Read the model definition and answer for the solid it produces. Units are mm, in the model's axes. A direction names the side the tool comes from. Round coordinates to 2 decimals unless told otherwise and drop trailing zeros. Order: outer loops, then holes, each group sorted by start corner. A loop starts at its lowest first (then second) coordinate and runs counter-clockwise, first axis right, second up. Notation, with made-up numbers: (9, -7) -> (15, -7) arc R31 ccw to (15, 22) -> close; hole circle Ø7 at (79.25, -36). An arc over 180 degrees is marked (long way). One line per item, written item: value. Start each with the question number.
1. Consider line 1 (X direction, y = -10.5, z = 4.25); line 2 (Y direction, x = -12, z = 5); line 3 (Z direction, x = -15, y = 9.75). Determine where each line is inside the solid, lowest interval first.
2. Section B-B (y = -10) is taken. Give the vertices of the cut face in (x, z).
3. Section A-A (z = 4.75) is taken. State how many separate pieces and enclosed holes the cut face has, then the cut area to 3 significant figures.
4. Section C-C (x = -8) is taken. Give the vertices of the cut face in (y, z).
5. Flat-ended cylindrical pins translate along their axes: pin 1 Ø3 at (y, z) = (-9, 1.5) entering from +X; pin 2 Ø8 at (x, y) = (4.5, -2) entering from +Z. Find the tip coordinate at first contact, or state that the pin passes through.
6. For faces 1 (the face through (0, 14, 1)), 2 (the face through (-15.1, 7.675, 7.3)), 3 (the face through (-13.3, 0, 1)), determine the directions among +Z, -Z, +X, -X, +Y, -Y from which every point of the face is accessible in a straight line to the end or side of a thin tool.
7. The mould has two halves that part along X. Classify faces 4 (the face through (13, -2.217, 1)), 5 (the face through (0, -14, 1)): released by +X, released by -X, zero draft, split by the parting line, or undercut.
from build123d import *

# Parameters (mm, degrees)
F0_W     = 30
F0_H     = 28
F1_DEPTH = 1.5
F3_DEPTH = 28
F4_W     = 1.3
F4_H     = 4
F5_DEPTH = 25
F6_W     = 41.33358
F6_H     = 15.079705
F7_DEPTH = 25


with BuildPart() as f1:
    # F0 (on Top) → F1 (new body)
    with BuildSketch(Plane.XY):
        Rectangle(F0_W, F0_H)
    extrude(amount=F1_DEPTH)

    # F2 (on face) → F3 (join)
    with BuildSketch(Plane.XZ.offset(14)):
        with BuildLine():
            ThreePointArc((-11.75963, 1.5), (-11.010384, 2.78526), (-10.75, 4.25))
            ThreePointArc((-10.75, 4.25), (-18.005204, 7.255204), (-15, 0))
            Line((-15, 0), (-15, 1.5))
            Line((-15, 1.5), (-11.75963, 1.5))
        make_face()
        with BuildLine():
            ThreePointArc((-12.25, 4.25), (-13.055456, 2.305456), (-15, 1.5))
            ThreePointArc((-15, 1.5), (-16.944544, 6.194544), (-12.25, 4.25))
        make_face(mode=Mode.SUBTRACT)
        with BuildLine():
            Line((15, 1.5), (15, 0))
            ThreePointArc((15, 0), (18.005204, 1.244796), (19.25, 4.25))
            ThreePointArc((19.25, 4.25), (13.53526, 8.239616), (11.75963, 1.5))
            Line((11.75963, 1.5), (15, 1.5))
        make_face()
        with BuildLine():
            ThreePointArc((17.75, 4.25), (16.944544, 2.305456), (15, 1.5))
            ThreePointArc((15, 1.5), (13.055456, 6.194544), (17.75, 4.25))
        make_face(mode=Mode.SUBTRACT)
        with BuildLine():
            Line((-15, 1.5), (-15, 0))
            ThreePointArc((-15, 0), (-13.214643, 0.393188), (-11.75963, 1.5))
            Line((-11.75963, 1.5), (-15, 1.5))
        make_face()
    extrude(amount=-F3_DEPTH)

    # F4 (on face) → F5 (cut)
    with BuildSketch(Plane.XY.offset(1.5)):
        with Locations((-12.65, -0.217311)):
            Rectangle(F4_W, F4_H)
        with Locations((12.65, -0.217311)):
            Rectangle(F4_W, F4_H)
    extrude(amount=-F5_DEPTH, mode=Mode.SUBTRACT)

    # F6 (on face) → F7 (cut)
    with BuildSketch(Plane.XY.offset(1.5)):
        with Locations((0.027121, 0.135609)):
            Rectangle(F6_W, F6_H)
    extrude(amount=F7_DEPTH, mode=Mode.SUBTRACT)


solid = f1.part
Answer:
1. line 1: -19.25 to -17.75, -12.25 to -10.75, 10.75 to 12.25, 17.75 to 19.25
1. line 2: -14 to -7.4, 7.68 to 14
1. line 3: 0 to 1.5, 7 to 8.5
2. outline: (-15, 0) -> (15, 0) arc R4.25 ccw (long way) to (11.76, 1.5) -> (-11.76, 1.5) arc R4.25 ccw (long way) to start; hole (-15, 1.5) arc R2.75 ccw to (-12.25, 4.25) arc R2.75 ccw (long way) to start; hole (15, 1.5) arc R2.75 ccw to (17.75, 4.25) arc R2.75 ccw (long way) to start
3. separate pieces: 8
3. enclosed holes: 0
3. area: 78.4 mm^2
4. outline: (-14, 0) -> (14, 0) -> (14, 1.5) -> (-14, 1.5) -> close
5. pin 1: x = 19.06
5. pin 2: z = 1.5
6. face 1: +Z, -Z, +X, -X, +Y
6. face 2: +Z, +X, -X
6. face 3: +Z, -Z
7. face 4: undercut
7. face 5: zero draft
